Can you work these out from the drawing? Everything is in mm from the part's minimum corner. Coordinates: 2 decimals unless noted, no trailing zeros. Loops run counter-clockwise (first coordinate to the right, second up) from the corner with the lowest first, then second, coordinate; pieces in that order, holes last.
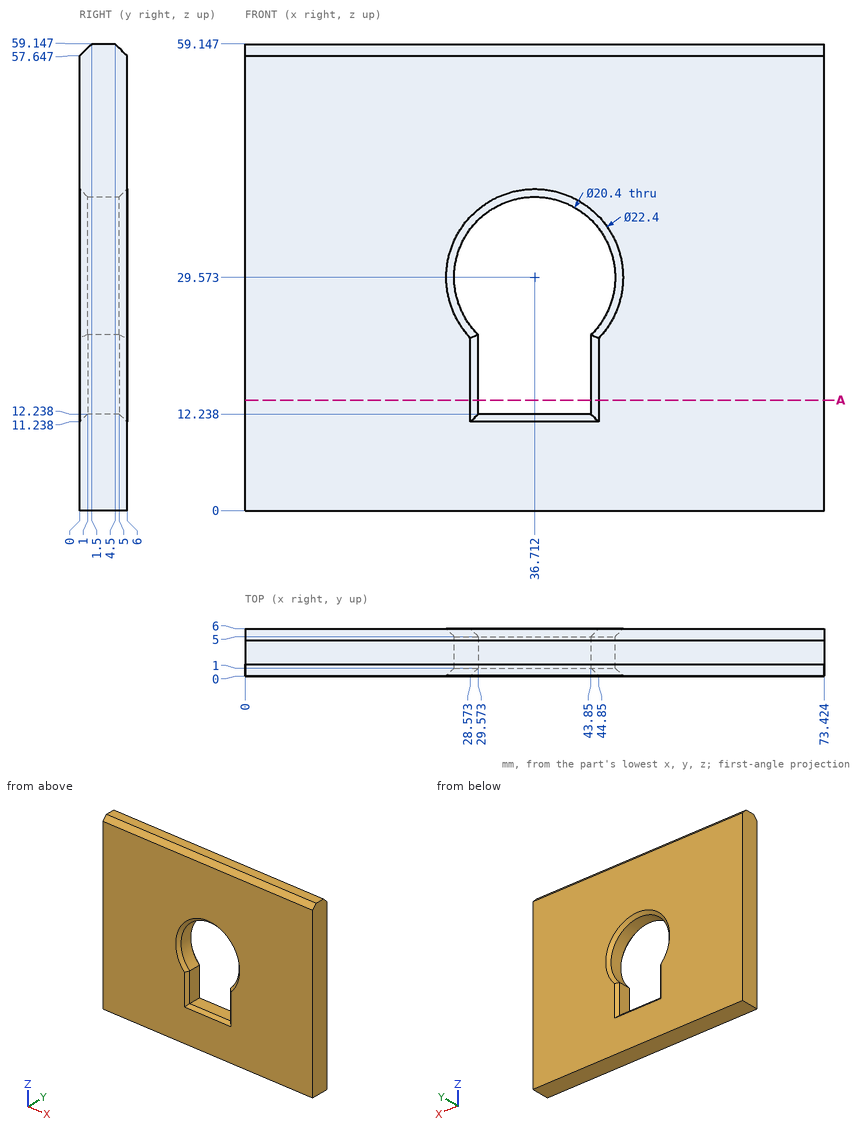
(1) For pin 1 (4 mm diameter, centred on x = 30.5, z = 35, fed in from -Y), with a flat end and sliding along its axis, tell me the tip position at first contact or that it passes through.
Answers:
pin 1: stops at y = 0.95
(2) I need wall thicknesses on probe 1 along X at (y, z) = (1.25, 30); probe 2 along Z at (x, y) = (29.5, 2.25) (1 decimal); probe 3 along Z at (x, y) = (39, 0.5) (1 decimal). Which ranges of each line are inside material? Lowest first, please.
Answers:
probe 1: x = 0 to 26.52, 46.9 to 73.42
probe 2: z = 0 to 22.4, 36.8 to 59.1
probe 3: z = 0 to 11.7, 40 to 58.1
(3) Imagine slicing it at A-A, the plane z = 14. Write out the boundary of the cut face in (x, y).
Answers:
outline: (0, 0) - (28.57, 0) - (29.57, 1) - (29.57, 5) - (28.57, 6) - (0, 6) - close; (43.85, 1) - (44.85, 0) - (73.42, 0) - (73.42, 6) - (44.85, 6) - (43.85, 5) - close
